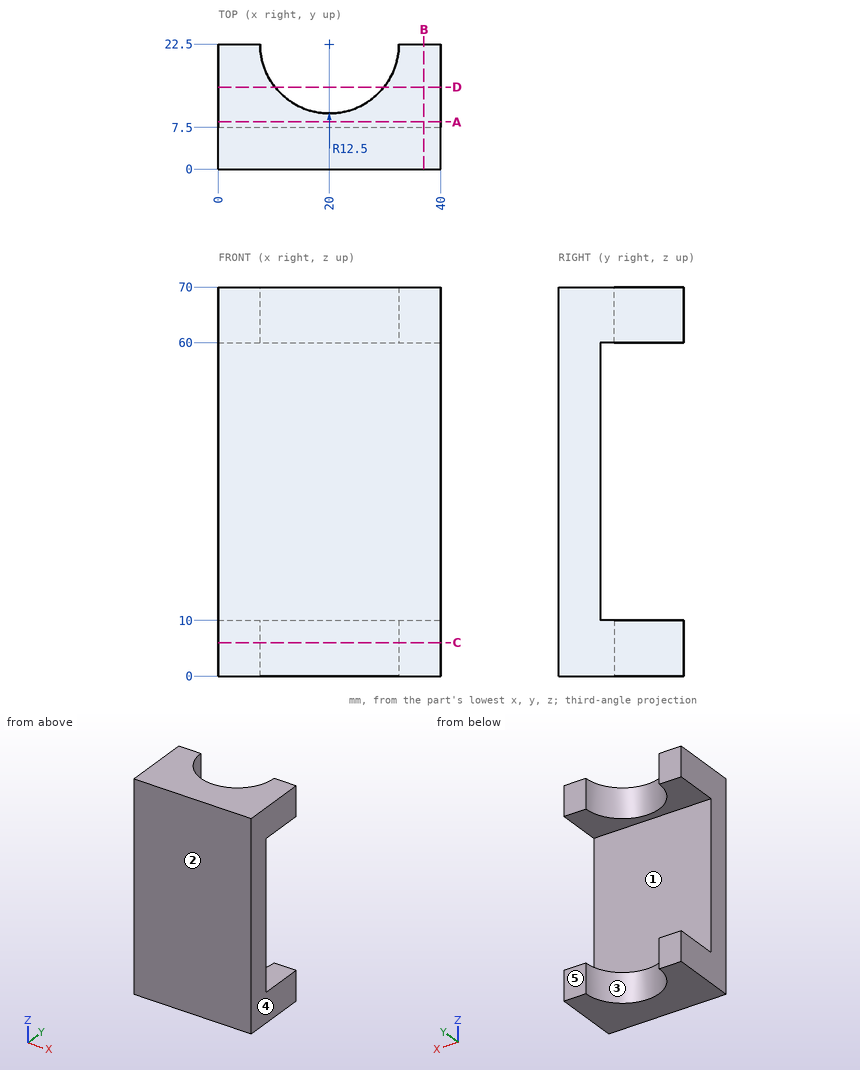
Here's the drawing with two shaded views (mm, measured from the low corner). I have some questions. A direction names the side the tool comes from. Coordinates: 2 decimals unless noted, no trailing zeros. Write each loop counter-clockwise with the first axis right and the second up, starting at its lowest first coordinate (ties: lowest second). Pieces come first, ordered by that corner, then holes.
Item 1: Will these pins go through, and if not, where does the flat tip stop? pin 1 (7.5 mm diameter, centred on x = 16, y = 17, fed in from +Z); pin 2 (4 mm diameter, centred on x = 25, z = 24, fed in from +Y); pin 3 (4 mm diameter, centred on x = 22.5, z = 10.5, fed in from +Y).
Item 2: If we mould it in two halves opening along X, with no side actions, what happens to the marked faces 3, 4 and 5? For each: +X half, -X half, draft (parallel to the pull), parting line (faces both ways), or undercut.
Item 3: I want a section at B-B on x = 37. Write out the boundary of the cut face in (y, z).
Item 4: If I drill on line 1 (Z direction, x = 32, y = 16.5); line 2 (Y direction, x = 3, z = 16); line 3 (X direction, y = 12.5, z = 61.5), over which ranges is the centre line in solid material (lowest first)?
Item 5: On a 3-axis mill with a long thin cutter (end or side, diameter ignored), from which of +Z, -Z, +X, -X, +Y, -Y can I reach the whole of each face in a straight line? I mean the marked faces 1 and 2. Say none if no direction works.
Item 6: I want a section at A-A on y = 8.5. Write out the boundary of the cut face in (x, z), and give its area (3 significant figures).
Item 7: I want a section at C-C on z = 6. Write out the boundary of the cut face in (x, y).
Item 8: I want a section at D-D on y = 14.75. Write out the boundary of the cut face in (x, z), and give its area (3 significant figures).
Findings below:
1. pin 1: passes through
1. pin 2: stops at y = 7.5
1. pin 3: stops at y = 10.81
2. face 3: undercut
2. face 4: +X half
2. face 5: draft
3. outline: (0, 0) - (22.5, 0) - (22.5, 10) - (7.5, 10) - (7.5, 60) - (22.5, 60) - (22.5, 70) - (0, 70) - close
4. line 1: z = 0 to 10, 60 to 70
4. line 2: y = 0 to 7.5
4. line 3: x = 0 to 12.5, 27.5 to 40
5. face 1: +X, -X, +Y
5. face 2: +Z, -Z, +X, -X, -Y
6. outline: (0, 0) - (40, 0) - (40, 10) - (0, 10) - close; (0, 60) - (40, 60) - (40, 70) - (0, 70) - close
6. area: 800 mm2
7. outline: (0, 0) - (40, 0) - (40, 22.5) - (32.5, 22.5) arc R12.5 cw to (7.5, 22.5) - (0, 22.5) - close
8. outline: (0, 0) - (10.19, 0) - (10.19, 10) - (0, 10) - close; (0, 60) - (10.19, 60) - (10.19, 70) - (0, 70) - close; (29.81, 0) - (40, 0) - (40, 10) - (29.81, 10) - close; (29.81, 60) - (40, 60) - (40, 70) - (29.81, 70) - close
8. area: 408 mm2
